Autodesk Inventor part; units mm, degrees
ref_plane "Work Plane1" through (-13.2583, 0, 13.2583) normal (-0.7071, 0, 0.7071) x (0, -1, 0)
ref_plane "YZ Plane" through (0, 0, 0) normal (1, 0, 0) x (0, 1, 0)
ref_plane "XZ Plane" through (0, 0, 0) normal (0, 1, 0) x (-1, 0, 0)
sketch "Sketch1" plane through (0, 0, 0) normal (0, 1, 0) x (-1, 0, 0)
  circle A0 centre (0, 0) radius 16.05
  circle A1 centre (0, 0) radius 18.75
  point P0 (18.75, 0)
  point P1 (13.2583, 13.2583)
  dimension "d0" = 32.1
  dimension "d4" = 45
  dimension "d9" = 2.7
extrude "Extrusion1" add sketch "Sketch1" along normal blind 6
ref_plane "Work Plane1" through (-13.2583, 0, 13.2583) normal (-0.7071, 0, 0.7071) x (0, -1, 0)
sketch "Sketch2" plane through (-13.2583, 0, 13.2583) normal (-0.7071, 0, 0.7071) x (0, -1, 0)
  circle A0 centre (-3, 0) radius 1.5
  circle A1 centre (-3, 0) radius 2.5
  point P0 (0, 0)
  dimension "d5" = 3
  dimension "d6" = 5
  dimension "d7" = 3
  dimension "d10" = 0
extrude "Extrusion2" add sketch "Sketch2" along normal mid plane 6
sketch "Sketch3" plane through (-15.3796, 3, 15.3796) normal (-0.7071, 0, 0.7071) x (0.7071, 0, 0.7071)
  circle A0 centre (0, 0) radius 1.5
  point P0 (0, -3)
extrude "Extrusion3" cut sketch "Sketch3" against normal blind 9.75
sketch "Sketch6" plane through (0, 0, 0) normal (0, -1, 0) x (1, 0, 0)
  line L0 (-17.4129, -27) -> (-9.4129, -27)
  line L1 (-9.4129, -27) -> (-9.4129, -13)
  line L2 (-9.4129, -13) -> (-17.4129, -13)
  line L3 (-17.4129, -13) -> (-17.4129, -27)
  circle A0 centre (0, 0) radius 16.05
  point P0 (-13.4129, -27)
  dimension "d15" = 14
  dimension "d16" = 8
  dimension "d34" = 13
extrude "Extrusion4" add sketch "Sketch6" along normal blind 8 contours L3 L2 L1 L0
sketch "Sketch7" plane through (-17.4129, 0, -27) normal (-1, 0, 0) x (0, 0, 1)
  line L0 (12, 0) -> (2, 0)
  line L1 (2, 0) -> (2, -6)
  line L2 (2, -6) -> (12, -6)
  line L3 (12, -6) -> (12, 0)
  line L4 (14, 0) -> (14, -8)
  line L5 (14, -8) -> (0, -8)
  point P0 (27, 0)
  dimension "d19" = 10
  dimension "d20" = 6
  dimension "d21" = 2
  dimension "d22" = 2
extrude "Extrusion5" cut sketch "Sketch7" against normal blind 10
sketch "Sketch8" plane through (0, 0, -13) normal (0, 0, 1) x (1, 0, 0)
  line L0 (-13.5116, 0) -> (-9.4129, 0)
  line L1 (-10.9129, 0) -> (-13.9129, 0)
  line L2 (-13.9129, 0) -> (-13.9129, -4)
  line L3 (-13.9129, -4) -> (-10.9129, -4)
  line L4 (-10.9129, -4) -> (-10.9129, 0)
  line L5 (-9.4129, 0) -> (-9.4129, -8)
  line L6 (-17.4129, -6) -> (-9.4129, -6)
  point P0 (0, 0)
  point P1 (-4, 0)
  dimension "d25" = 1.5
  dimension "d26" = 3
  dimension "d27" = 2
extrude "Extrusion6" cut sketch "Sketch8" against normal blind 15.25
sketch "Sketch9" plane through (-9.4129, -8, -27) normal (0, 0, -1) x (-1, 0, 0)
  line L0 (6.6371, 8) -> (-25.4629, 8)
  line L1 (0, 8) -> (8, 8)
  line L2 (8, 8) -> (8, 14)
  line L3 (8, 14) -> (0, 14)
  line L4 (0, 14) -> (0, 8)
  point P0 (-9.4129, 8)
  dimension "d30" = 6
extrude "Extrusion7" add sketch "Sketch9" against normal blind 20.5
sketch "Sketch10" plane through (0, 0, 0) normal (0, -1, 0) x (1, 0, 0)
  circle A0 centre (0, 0) radius 16.05
  arc A1 (-9.4129, -13) -> (-14.6749, -6.5) centre (0, 0) ccw
extrude "Extrusion8" cut sketch "Sketch10" against normal blind 12.5
fillet "Fillet2" radius 2.5 1 edges at (-9.4129, 3, -16.216)
properties part number "DC_Ring"
The model under review builds one solid part; all positions refer to its coordinate system, in mm. A direction names the side the tool comes from. Round coordinates to 2 decimals unless told otherwise and drop trailing zeros. Loops run counter-clockwise (first coordinate to the right, second up) from the corner with the lowest first, then second, coordinate; pieces in that order, holes last. Notation, with made-up numbers: M 9,-28.75 L 17,-28.75 A26 ccw 17,-3.75 Z; hole C -27,-37.75 d11. An arc over 180 degrees is marked long. Answer as a JSON object with one key per item and string values.
(1) To check wall thickness, follow line 1 along Z through (x, y) = (0, 2.75); line 2 along X through (y, z) = (0.75, -10.5). State the ranges of each line that lie inside material, in increasing order.
Resolved:
{"line 1": "-18.75 to -16.05, 16.05 to 18.75", "line 2": "-17.41 to -12.14, 12.14 to 15.53"}
(2) Draft analysis for pull direction X (two halves, no side actions). For faces 1 (the flat face through (-16.53, 2.48, 14.23)), 2 (the flat face through (-13, -6, -20)), 3 (the flat face through (-13.913, -2, -14)), state which applies: released by +X, released by -X, zero draft, split by the parting line, or undercut.
Resolved:
{"face 1": "released by -X", "face 2": "zero draft", "face 3": "undercut"}
(3) Take a section at B-B on x = 0. Give the boundary of the cut face in (y, z), and give its area (3 significant figures).
Resolved:
{"outline": "M 0,-18.75 L 6,-18.75 L 6,-16.05 L 0,-16.05 Z; M 0,16.05 L 6,16.05 L 6,18.75 L 0,18.75 Z", "area": "32.4 mm²"}
(4) Clearance check with flat-ended pins moving along their axes: P1, Ø0.6, axis at y = -2.5, z = -26.5, coming from the -X side; P2, Ø6.5, axis at x = -12, y = -5.5, coming from the +Z side; P3, Ø3, axis at x = -13.5, z = 1, coming from the -Y side; P4, Ø6, axis at x = -6.5, y = 1.5, coming from the +Z side. State where each tip first meets the part, or that it passes through.
Resolved:
{"P1": "x = -17.41", "P2": "z = -13", "P3": "through", "P4": "z = 18.42"}
(5) Tool access review of faces 4 (the flat face through (-9.413, 1, -22)), 5 (the flat face through (-13, -5, -13)), 6 (the flat face through (-10.913, -2, -26)), 7 (the flat face through (-14.4, -3, -15)): name each direction out of +Z, -Z, +X, -X, +Y, -Y from which nothing blocks a thin tool from reaching the whole face with its end or side.
Resolved:
{"face 4": "-Z, +X, -Y", "face 5": "+Z, +X, -X, -Y", "face 6": "+Z, -Z", "face 7": "+X, -X"}
(6) Take a section at A-A on z = -21.5. Give the boundary of the cut face in (x, y).
Resolved:
{"outline": "M -17.41,-8 L -9.41,-8 L -9.41,-6 L -17.41,-6 Z; M -17.41,0 L -9.41,0 L -9.41,6 L -17.41,6 Z"}
(7) Take a section at C-C on y = -6.5. Give the boundary of the cut face in (x, z), and give its area (3 significant figures).
Resolved:
{"outline": "M -17.41,-27 L -9.41,-27 L -9.41,-13 L -17.41,-13 Z", "area": "112 mm²"}
